Here's how the part is built. I have some questions about the finished solid (model axes, mm). Give positions to 0.01 mm unless a question says otherwise; leave off trailing zeros. Write each loop counter-clockwise with the first axis right and the second up, starting at its lowest first coordinate (ties: lowest second). Pieces come first, ordered by that corner, then holes. Notation, with made-up numbers: (-12.5, -38.75) -> (31.5, -38.75) arc R18 cw to (31.5, -23.75) -> close; hole circle Ø8 at (55, -28). An arc over 180 degrees is marked (long way). Use CSV: the item, a comma, the result in double quotes. Start each with the question number.
(1) Suppose I cut it at D-D on y = -86. List the corners of the cut face in (x, z) for me, plus the area to 3 significant figures.
(2) I need wall thicknesses on L1, parallel to Y at x = -169.5, z = 320.5; L2, parallel to X at y = -203, z = 142; L3, parallel to Z at x = 75, y = -84. Which ranges of each line are inside material? Lowest first, please. Write a range as [from, to].
(3) Suppose I cut it at C-C on x = -147.5. List the corners of the cut face in (y, z) for me, plus the area to 3 significant figures.
(4) For pin 1 Ø2 at (x, z) = (2.5, 265.5) entering from -Y; pin 2 Ø2 at (x, z) = (-105, 309.5) entering from +Y; pin 3 Ø4 at (x, z) = (168, 285.5) entering from -Y, each with a flat end and sliding along its axis, tell me the tip position at first contact or that it passes through.
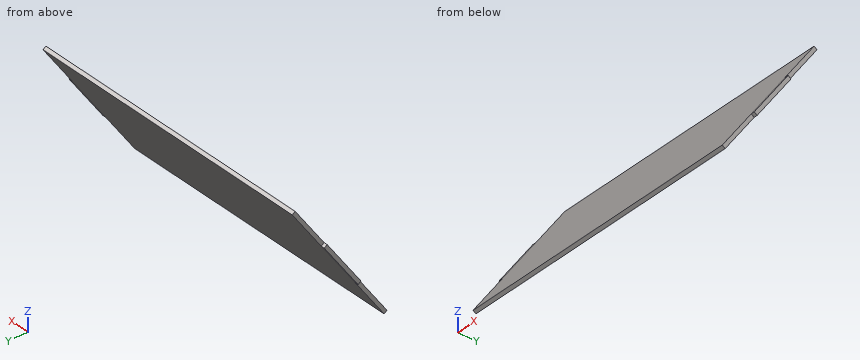
from build123d import *

# Parameters (mm, degrees)
PAD012_DEPTH = 250
SKETCH023_W  = 100
SKETCH023_H  = 6
PAD015_DEPTH = 6


with BuildPart() as part:
    # Sketch020 → Pad012 (new body, symmetric)
    with BuildSketch(Plane.YZ):
        Polygon((-222, 120), (-66.553927, 342), (-61.639014, 338.558541), (-217.085088, 116.558541), align=None)
    extrude(amount=PAD012_DEPTH, both=True)

    # Sketch023 (on Face1 of Pad012) → Pad015 (join)
    with BuildSketch(Plane(origin=(0, -205.345793, 143.784672), x_dir=(0, -0.573576, -0.819152), z_dir=(0, -0.819152, 0.573576))):
        with Locations((-106.470256, -253)):
            Rectangle(SKETCH023_W, SKETCH023_H)
    pad015 = extrude(amount=-PAD015_DEPTH)

    # Mirrored001: Pad015 across YZ
    add(pad015.mirror(Plane.YZ))


solid = part.part
Geometry says:
1,outline,"(-250, 303.77) -> (250, 303.77) -> (250, 314.23) -> (-250, 314.23) -> close"
1,area,"5,230 mm²"
2,L1,"[-81.61, -74.28]"
2,L2,"[-250, 250]"
2,L3,"[306.62, 317.08]"
3,outline,"(-222, 120) -> (-217.09, 116.56) -> (-61.64, 338.56) -> (-66.55, 342) -> close"
3,area,"1,630 mm²"
4,pin 1,"y = -120.82"
4,pin 2,"y = -81.29"
4,pin 3,"y = -107.52"
